Here's how the part is built. I have some questions about the finished solid (model axes, mm). Face numbers are marked on the shaded views. Coordinates: 2 decimals unless noted, no trailing zeros. Order: outer loops, then holes, each group sorted by start corner. A loop starts at its lowest first (then second) coordinate and runs counter-clockwise, first axis right, second up. Notation, with made-up numbers: M 29.5,-19 L 87.5,-19 A16 ccw 87.5,-12 Z; hole C -18.75,74 d3. An arc over 180 degrees is marked long. Answer as CSV lines item,"result". Start each with the question number.
```python
from build123d import *

# Parameters (mm, degrees)
SKETCH1_R           = 1.75
SKETCH1_R_2         = 3
BOSS_EXTRUDE1_DEPTH = 6
SKETCH2_R           = 3.5
CUT_EXTRUDE1_DEPTH  = 3


with BuildPart() as part:
    # Sketch1 → Boss-Extrude1 (new body)
    with BuildSketch(Plane(origin=(0, 0, 0), x_dir=(1, 0, 0), z_dir=(0, 1, 0))):
        with BuildLine():
            Line((1.176696811, -5.883484054), (-48.823303189, -15.883484054))
            ThreePointArc((-48.823303189, -15.883484054), (-55.883484054, -11.176696811), (-51.176696811, -4.116515946))
            Line((-51.176696811, -4.116515946), (-1.176696811, 5.883484054))
            ThreePointArc((-1.176696811, 5.883484054), (5.883484054, 1.176696811), (1.176696811, -5.883484054))
        make_face()
        with Locations(Location((0, 0, 0), (0, 0, 270))):
            Circle(SKETCH1_R, mode=Mode.SUBTRACT)
        with Locations(Location((-50, -10, 0), (0, 0, 270))):
            Circle(SKETCH1_R_2, mode=Mode.SUBTRACT)
    extrude(amount=BOSS_EXTRUDE1_DEPTH)

    # Sketch2 → Cut-Extrude1 (cut)
    with BuildSketch(Plane(origin=(0, 6, 0), x_dir=(1, 0, 0), z_dir=(0, 1, 0))):
        with Locations(Location((0, 0, 0), (0, 0, 270))):
            Circle(SKETCH2_R)
    extrude(amount=-CUT_EXTRUDE1_DEPTH, mode=Mode.SUBTRACT)


solid = part.part
```
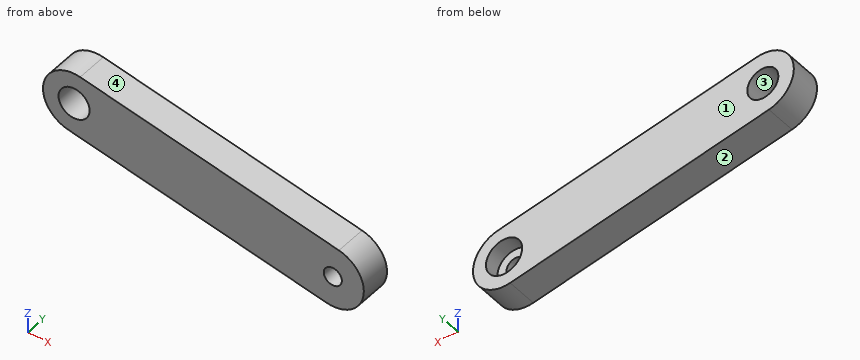
1) If we mould it in two halves opening along X, with no side actions, what happens to the marked faces 1, 2, 3 and 4? For each: released by +X, released by -X, zero draft, split by the parting line, or undercut.
2) Will these pins go through, and if not, where does the flat tip stop? pin 1 Ø1.5 at (x, y) = (-29.5, 5) entering from -Z; pin 2 Ø3.5 at (x, z) = (1, -1) entering from +Y; pin 3 Ø1 at (x, y) = (-13, 2) entering from +Z.
3) Suppose I cut it at C-C on z = 10. Please give me the cut outline in (x, y), plus the area to 3 significant figures.
4) Suppose I cut it at D-D on z = -2.5. Please give me the cut outline in (x, y).
5) Suppose I cut it at B-B on x = 0. Please give me the cut outline in (y, z).
6) I need wall thicknesses on line 1 (Y direction, x = 2, z = -0.75); line 2 (Z direction, x = 0, y = 2.2); line 3 (Z direction, x = -4, y = 5.75). Which ranges of each line are inside material? Lowest first, please. Write a range as [from, to].
Output:
1,face 1,"zero draft"
1,face 2,"released by -X"
1,face 3,"undercut"
1,face 4,"released by +X"
2,pin 1,"z = -0.37"
2,pin 2,"y = 3"
2,pin 3,"z = 8.82"
3,outline,"M -56,0 L -53,0 L -53,6 L -56,6 Z; M -47,0 L -19.41,0 L -19.41,6 L -47,6 Z"
3,area,"184 mm²"
4,outline,"M -18.09,0 L 5.45,0 L 5.45,6 L 2.45,6 L 2.45,3 L -2.45,3 L -2.45,6 L -18.09,6 Z"
5,outline,"M 0,-6 L 6,-6 L 6,-3.5 L 3,-3.5 L 3,-1.75 L 0,-1.75 Z; M 0,1.75 L 3,1.75 L 3,3.5 L 6,3.5 L 6,6.12 L 0,6.12 Z"
6,line 1,"[0, 3]"
6,line 2,"[-6, -1.75], [1.75, 6.12]"
6,line 3,"[-5.32, 6.92]"
